from build123d import *

# Parameters (mm, degrees)
SKETCH1_R               = 47.7
SKETCH1_R_2             = 35
BOSS_EXTRUDE1_DEPTH     = 76.2
CUT_EXTRUDE1_DEPTH      = 1
CUT_EXTRUDE1_DEPTH_BACK = 77.2
BOSS_EXTRUDE2_DEPTH     = 76.2
BOSS_EXTRUDE4_DEPTH     = 76.2
FILLET2_R               = 12.7
SKETCH6_W               = 40.64
SKETCH6_H               = 65.287260423
CUT_EXTRUDE3_DEPTH      = 101.6
CUT_EXTRUDE4_START      = -6.0800001
SKETCH7_R               = 2.5
CUT_EXTRUDE4_DEPTH      = 74.907260623
LPATTERN1_COUNT         = 3
LPATTERN1_PITCH         = 11.43
BOSS_EXTRUDE5_DEPTH     = 76.2
FILLET3_R               = 12.7
SKETCH8_W               = 40.64
SKETCH8_H               = 65.287260423
CUT_EXTRUDE5_DEPTH      = 76.2
CUT_EXTRUDE6_START      = -6.0800001
SKETCH9_R               = 2.5
CUT_EXTRUDE6_DEPTH      = 74.907260623
LPATTERN2_COUNT         = 3
LPATTERN2_PITCH         = 12.62


with BuildPart() as part:
    # Sketch1 → Boss-Extrude1 (new body)
    with BuildSketch(Plane.XY):
        Circle(SKETCH1_R)
        Circle(SKETCH1_R_2, mode=Mode.SUBTRACT)
    extrude(amount=BOSS_EXTRUDE1_DEPTH)

    # Sketch2 → Cut-Extrude1 (cut, two sides)
    with BuildSketch(Plane.XY.offset(76.2)) as cut_extrude1_sk:
        Polygon((-285.983619069, 0), (-50.977699953, 0), (54.190264056, 0), (289.196183172, 0), (289.196183172, 470.011838232), (-285.983619069, 470.011838232), align=None)
    extrude(amount=CUT_EXTRUDE1_DEPTH, mode=Mode.SUBTRACT)
    extrude(cut_extrude1_sk.sketch, amount=-CUT_EXTRUDE1_DEPTH_BACK, mode=Mode.SUBTRACT)

    # Sketch3 → Boss-Extrude2 (add)
    with BuildSketch(Plane(origin=(0, 0, 0), x_dir=(-1, 0, 0), z_dir=(0, 0, -1))):
        with BuildLine():
            ThreePointArc((-4.283714166, -47.507260423), (-35.210958278, -32.178850463), (-47.7, 0))
            Line((-47.7, 0), (-47.7, -47.507260423))
            Line((-47.7, -47.507260423), (-4.283714166, -47.507260423))
        make_face()
        with BuildLine():
            Line((47.7, -47.507260423), (47.7, 0))
            ThreePointArc((47.7, 0), (35.210958278, -32.178850463), (4.283714166, -47.507260423))
            Line((4.283714166, -47.507260423), (47.7, -47.507260423))
        make_face()
        with BuildLine():
            Line((-4.283714166, -47.507260423), (-47.7, -47.507260423))
            Line((-47.7, -47.507260423), (-47.7, -72.907260423))
            Line((-47.7, -72.907260423), (47.7, -72.907260423))
            Line((47.7, -72.907260423), (47.7, -47.507260423))
            Line((47.7, -47.507260423), (4.283714166, -47.507260423))
            ThreePointArc((4.283714166, -47.507260423), (0, -47.7), (-4.283714166, -47.507260423))
        make_face()
    extrude(amount=-BOSS_EXTRUDE2_DEPTH)

    # Sketch5 → Boss-Extrude4 (add)
    with BuildSketch(Plane(origin=(0, 0, 0), x_dir=(-1, 0, 0), z_dir=(0, 0, -1))):
        Polygon((-47.7, 0), (-47.7, -72.907260423), (-79.45, -72.907260423), align=None)
    extrude(amount=-BOSS_EXTRUDE4_DEPTH)

    # Fillet2
    fillet2_edges = [part.edges().sort_by_distance(p)[0] for p in [
        (63.575, -36.453630212, 0),
        (63.575, -36.453630212, 76.2),
    ]]
    fillet(fillet2_edges, radius=FILLET2_R)

    # Sketch6 → Cut-Extrude3 (cut)
    with BuildSketch(Plane(origin=(47.7, 0, 0), x_dir=(0, 0, -1), z_dir=(1, 0, 0))):
        with Locations((-38.1, -35.183630212)):
            Rectangle(SKETCH6_W, SKETCH6_H)
    extrude(amount=CUT_EXTRUDE3_DEPTH, mode=Mode.SUBTRACT)

    # Sketch7 → Cut-Extrude4 (cut)
    with BuildSketch(Plane(origin=(0, -67.827260423, 0), x_dir=(1, 0, 0), z_dir=(0, 1, 0)).offset(CUT_EXTRUDE4_START)):
        with Locations((61.997737475, -50.8)):
            Circle(SKETCH7_R)
    cut_extrude4 = extrude(amount=CUT_EXTRUDE4_DEPTH, mode=Mode.SUBTRACT)

    # LPattern1: Cut-Extrude4 ×3
    with Locations(*[(0, 0, -i * LPATTERN1_PITCH) for i in range(1, LPATTERN1_COUNT)]):
        add(cut_extrude4, mode=Mode.SUBTRACT)

    # Sketch4 → Boss-Extrude5 (add)
    with BuildSketch(Plane(origin=(0, 0, 0), x_dir=(-1, 0, 0), z_dir=(0, 0, -1))):
        Polygon((47.7, 0), (47.7, -72.907260423), (79.45, -72.907260423), align=None)
    extrude(amount=-BOSS_EXTRUDE5_DEPTH)

    # Fillet3
    fillet3_edges = [part.edges().sort_by_distance(p)[0] for p in [
        (-63.575, -36.453630212, 0),
        (-63.575, -36.453630212, 76.2),
    ]]
    fillet(fillet3_edges, radius=FILLET3_R)

    # Sketch8 → Cut-Extrude5 (cut)
    with BuildSketch(Plane.ZY.offset(47.7)):
        with Locations((38.1, -35.183630212)):
            Rectangle(SKETCH8_W, SKETCH8_H)
    extrude(amount=CUT_EXTRUDE5_DEPTH, mode=Mode.SUBTRACT)

    # Sketch9 → Cut-Extrude6 (cut)
    with BuildSketch(Plane(origin=(0, -67.827260423, 0), x_dir=(1, 0, 0), z_dir=(0, 1, 0)).offset(CUT_EXTRUDE6_START)):
        with Locations((-61.997737475, -50.8)):
            Circle(SKETCH9_R)
    cut_extrude6 = extrude(amount=CUT_EXTRUDE6_DEPTH, mode=Mode.SUBTRACT)

    # LPattern2: Cut-Extrude6 ×3
    with Locations(*[(0, 0, -i * LPATTERN2_PITCH) for i in range(1, LPATTERN2_COUNT)]):
        add(cut_extrude6, mode=Mode.SUBTRACT)


solid = part.part
CAD build for the part. Positions are in the model's coordinates, mm. Coordinates: 2 decimals unless noted, no trailing zeros. Loops run counter-clockwise (first coordinate to the right, second up) from the corner with the lowest first, then second, coordinate; pieces in that order, holes last. Notation, with made-up numbers: (77.5, 56.5) -> (99.5, 56.5) arc R27 ccw to (99.5, 91.5) -> close; hole circle Ø4 at (27.5, -27). An arc over 180 degrees is marked (long way). One line per item, written item: value.
1. Slice it at B-B on x = 0. Write the cut outline in (y, z).
Answers:
outline: (-72.91, 0) -> (-35, 0) -> (-35, 76.2) -> (-72.91, 76.2) -> close
2. Pull direction X, two halves, no side cores. Call faces 1 (the face through (-58.82, -35.11, 72.58)), 2 (the face through (59, -43, 58.42)), 3 (the face through (-0.77, -34.99, 37.57)), 4 (the face through (66, -42.02, 58.68)): pulls with the +X half, pulls with the -X half, needs draft (parallel to the pull), parting line crosses it, or undercut.
Answers:
face 1: pulls with the -X half
face 2: needs draft
face 3: undercut
face 4: pulls with the +X half
3. Slice it at C-C on z = 11. Write the cut outline in (x, y).
Answers:
outline: (-79.33, -72.91) -> (79.33, -72.91) -> (47.58, 0) -> (35, 0) arc R35 cw to (-35, 0) -> (-47.58, 0) -> close
4. Drill centre lines: line 1 (Z direction, x = 60, y = -58.5); line 2 (X direction, y = -69, z = 38); line 3 (X direction, y = -71, z = 38). Where is each one in solid material? Low to high. Write a range as [from, to].
Answers:
line 1: z = [0.02, 17.78], [58.42, 76.18]
line 2: x = [-77.75, -64.49], [-59.5, 59.91], [64.09, 77.75]
line 3: x = [-78.62, -64.49], [-59.5, 59.91], [64.09, 78.62]
5. Flat gauge pins, fed straight in: P1, Ø5, axis at y = -33, z = 48.5, coming from the +X side; P2, Ø23.5, axis at x = 59.5, z = 39.5, coming from the +Y side; P3, Ø23.5, axis at x = 59, y = -24.5, coming from the +Z side. Where does each tip first touch, or does it go through?
Answers:
P1: stops at x = 47.7
P2: stops at y = -0.11
P3: stops at z = 76.11
6. Slice it at A-A on z = 50.8. Write the cut outline in (x, y), and give its area (3 significant figures).
Answers:
outline: (-79.45, -72.91) -> (-64.5, -72.91) -> (-64.5, -67.83) -> (-77.24, -67.83) -> close; (-59.5, -72.91) -> (59.5, -72.91) -> (59.5, -67.83) -> (47.7, -67.83) -> (47.7, -2.54) -> (48.81, -2.54) -> (47.7, 0) -> (35, 0) arc R35 cw to (-35, 0) -> (-47.7, 0) -> (-48.81, -2.54) -> (-47.7, -2.54) -> (-47.7, -67.83) -> (-59.5, -67.83) -> close; (64.5, -72.91) -> (79.45, -72.91) -> (77.24, -67.83) -> (64.5, -67.83) -> close
area: 5,290 mm^2
